Input: part model. Units: mm. Frame: model coordinates. Face numbers are marked on the shaded views. A direction names the side the tool comes from. Coordinates: 2 decimals unless noted, no trailing zeros. Order: outer loops, then holes, each group sorted by start corner. A loop starts at its lowest first (then second) coordinate and runs counter-clockwise, first axis right, second up. Notation, with made-up numbers: (66, 52.5) -> (116, 52.5) arc R31 cw to (116, 80.5) -> close; hole circle Ø7 at (-14.75, 62). An arc over 180 degrees is marked (long way). Answer as CSV lines item,"result".
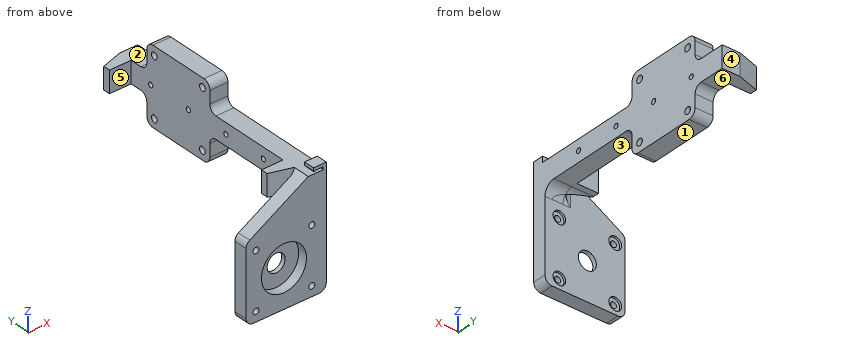
from build123d import *

# Parameters (mm, degrees)
SKETCH1_W           = 42
SKETCH1_H           = 42
SKETCH1_R           = 1.9
BOSS_EXTRUDE1_DEPTH = 10
SKETCH2_W           = 12
SKETCH2_H           = 118
BOSS_EXTRUDE2_DEPTH = 10
SKETCH3_W           = 12
SKETCH3_H           = 3.75
BOSS_EXTRUDE3_DEPTH = 12
CHAMFER1_SIZE       = 3.75
CHAMFER1_SIZE_2     = 12.265697319
SKETCH4_R           = 1.375
CUT_EXTRUDE1_DEPTH  = 12
SKETCH5_W           = 42
SKETCH5_H           = 42
SKETCH5_R           = 1.65
SKETCH5_R_2         = 5
BOSS_EXTRUDE4_DEPTH = 7.5
SKETCH6_R           = 12.5
CUT_EXTRUDE2_DEPTH  = 5.2
FILLET1_R           = 4
FILLET2_R           = 6
SKETCH8_R           = 3.5
CUT_EXTRUDE4_DEPTH  = 1.2
BOSS_EXTRUDE7_DEPTH = 6


with BuildPart() as part:
    # Sketch1 → Boss-Extrude1 (new body)
    with BuildSketch(Plane(origin=(0, 0, 0), x_dir=(0, 0, -1), z_dir=(1, 0, 0))):
        Rectangle(SKETCH1_W, SKETCH1_H)
        with Locations((16, -16)):
            Circle(SKETCH1_R, mode=Mode.SUBTRACT)
        with Locations((-16, -16)):
            Circle(SKETCH1_R, mode=Mode.SUBTRACT)
        with Locations((-16, 16)):
            Circle(SKETCH1_R, mode=Mode.SUBTRACT)
        with Locations((16, 16)):
            Circle(SKETCH1_R, mode=Mode.SUBTRACT)
    extrude(amount=BOSS_EXTRUDE1_DEPTH)

    # Sketch2 → Boss-Extrude2 (add)
    with BuildSketch(Plane.ZY):
        with Locations((0, -20)):
            Rectangle(SKETCH2_W, SKETCH2_H)
    extrude(amount=-BOSS_EXTRUDE2_DEPTH)

    # Sketch3 → Boss-Extrude3 (add)
    with BuildSketch(Plane.ZY):
        with Locations((0, 33.375)):
            Rectangle(SKETCH3_W, SKETCH3_H)
        with Locations((0, -71.575)):
            Rectangle(SKETCH3_W, SKETCH3_H)
    extrude(amount=BOSS_EXTRUDE3_DEPTH)

    # Chamfer1
    # the kernel refuses this chamfer: 12.265697319, 3.75 mm, written as the material it adds along each edge
    with BuildSketch(Plane(origin=(0, 35.25, -6), x_dir=(0.11964200288050787, 0.9928170985366542, 0), z_dir=(0, 0, 1))) as chamfer1_piece_1_section:
        Polygon((CHAMFER1_SIZE * 0.992817098537, CHAMFER1_SIZE * 0.119642002881), (-CHAMFER1_SIZE_2 * 0.119642002884, CHAMFER1_SIZE_2 * 0.992817098562), (0, 0), align=None)
    chamfer1_piece_1 = extrude(amount=12, mode=Mode.PRIVATE)
    chamfer1_piece_1 = split(chamfer1_piece_1, bisect_by=Plane(origin=(-4.172539525, 39, 0), z_dir=(0, -1, 0)), keep=Keep.TOP, mode=Mode.PRIVATE)
    chamfer1_piece_1 = split(chamfer1_piece_1, bisect_by=Plane(origin=(-12, 36.383581674, 0), z_dir=(1, 0, 0)), keep=Keep.TOP, mode=Mode.PRIVATE)
    add(chamfer1_piece_1)
    with BuildSketch(Plane(origin=(0, -73.45, -6), x_dir=(0.11964200288050787, -0.9928170985366542, 0), z_dir=(0, 0, 1))) as chamfer1_piece_2_section:
        Polygon((CHAMFER1_SIZE * 0.992817098537, -CHAMFER1_SIZE * 0.119642002881), (-CHAMFER1_SIZE_2 * 0.119642002884, -CHAMFER1_SIZE_2 * 0.992817098562), (0, 0), align=None)
    chamfer1_piece_2 = extrude(amount=12, mode=Mode.PRIVATE)
    chamfer1_piece_2 = split(chamfer1_piece_2, bisect_by=Plane(origin=(-12, -74.58994207, 0), z_dir=(1, 0, 0)), keep=Keep.TOP, mode=Mode.PRIVATE)
    add(chamfer1_piece_2)

    # Sketch4 → Cut-Extrude1 (cut)
    with BuildSketch(Plane.ZY):
        with Locations((0, 18.4)):
            Circle(SKETCH4_R)
        with Locations((0, -6.6)):
            Circle(SKETCH4_R)
        with Locations((0, -31.6)):
            Circle(SKETCH4_R)
        with Locations((0, -56.6)):
            Circle(SKETCH4_R)
    extrude(amount=-CUT_EXTRUDE1_DEPTH, mode=Mode.SUBTRACT)

    # Sketch5 → Boss-Extrude4 (add)
    # profile 1 of 2: a face of its own
    with BuildSketch(Plane.XZ.offset(79)):
        Polygon((10, -56), (10, 6), (0, 6), (-34.5, -14), (7.5, -14), (7.5, -56), align=None)
    # profile 2 of 2: a face of its own
    with BuildSketch(Plane.XZ.offset(79)):
        with Locations((-13.5, -35)):
            Rectangle(SKETCH5_W, SKETCH5_H)
        with Locations(Location((-29, -50.5, 0), (0, 0, 270))):
            Circle(SKETCH5_R, mode=Mode.SUBTRACT)
        with Locations(Location((-13.5, -35, 0), (0, 0, 270))):
            Circle(SKETCH5_R_2, mode=Mode.SUBTRACT)
        with Locations(Location((2, -50.5, 0), (0, 0, 270))):
            Circle(SKETCH5_R, mode=Mode.SUBTRACT)
        with Locations(Location((-29, -19.5, 0), (0, 0, 270))):
            Circle(SKETCH5_R, mode=Mode.SUBTRACT)
        with Locations(Location((2, -19.5, 0), (0, 0, 270))):
            Circle(SKETCH5_R, mode=Mode.SUBTRACT)
    extrude(amount=BOSS_EXTRUDE4_DEPTH)

    # Sketch6 → Cut-Extrude2 (cut)
    with BuildSketch(Plane.XZ.offset(86.5)):
        with Locations(Location((-13.5, -35, 0), (0, 0, 270))):
            Circle(SKETCH6_R)
    extrude(amount=-CUT_EXTRUDE2_DEPTH, mode=Mode.SUBTRACT)

    # Fillet1
    fillet1_edges = [part.edges().sort_by_distance(p)[0] for p in [
        (-34.5, -82.75, -56),
        (10, -82.75, -56),
        (-34.5, -82.75, -14),
        (5, -21, 6),
        (5, -21, -6),
        (5, 21, -6),
        (5, 21, 6),
        (5, -21, -21),
        (5, -21, 21),
        (5, 21, 21),
        (5, 21, -21),
    ]]
    fillet(fillet1_edges, radius=FILLET1_R)

    # Fillet2
    # the kernel refuses this fillet: 6 mm, written as the material it adds along each edge
    with BuildSketch(Plane(origin=(0, -79, -6), x_dir=(0, 1, 0), z_dir=(1, 0, 0))) as fillet2_piece_1_section:
        with BuildLine():
            CenterArc((FILLET2_R, -FILLET2_R), FILLET2_R, 90, 90)
            Line((0, -FILLET2_R), (-FILLET2_R * 0.02, -FILLET2_R))
            Line((-FILLET2_R * 0.02, -FILLET2_R), (-FILLET2_R * 0.02, FILLET2_R * 0.02))
            Line((-FILLET2_R * 0.02, FILLET2_R * 0.02), (FILLET2_R, FILLET2_R * 0.02))
            Line((FILLET2_R, FILLET2_R * 0.02), (FILLET2_R, 0))
        make_face()
    fillet2_piece_1 = extrude(amount=10, mode=Mode.PRIVATE)
    fillet2_piece_1 = split(fillet2_piece_1, bisect_by=Plane(origin=(2.499298027, -77.964112089, -8.062690797), z_dir=(-0.29237170472287155, -0.9563047559629945, 0)), keep=Keep.TOP, mode=Mode.PRIVATE)
    add(fillet2_piece_1)
    with BuildSketch(Plane(origin=(-15, -79, -6), x_dir=(0, 1, 0), z_dir=(1, 0, 0))) as fillet2_piece_2_section:
        with BuildLine():
            CenterArc((FILLET2_R, -FILLET2_R), FILLET2_R, 90, 90)
            Line((0, -FILLET2_R), (-FILLET2_R * 0.02, -FILLET2_R))
            Line((-FILLET2_R * 0.02, -FILLET2_R), (-FILLET2_R * 0.02, FILLET2_R * 0.02))
            Line((-FILLET2_R * 0.02, FILLET2_R * 0.02), (FILLET2_R, FILLET2_R * 0.02))
            Line((FILLET2_R, FILLET2_R * 0.02), (FILLET2_R, 0))
        make_face()
    fillet2_piece_2 = extrude(amount=25, mode=Mode.PRIVATE)
    fillet2_piece_2 = split(fillet2_piece_2, bisect_by=Plane(origin=(-12, -75.195203729, -6.203668613), z_dir=(1, 0, 0)), keep=Keep.TOP, mode=Mode.PRIVATE)
    fillet2_piece_2 = split(fillet2_piece_2, bisect_by=Plane(origin=(-3.530108064, -76.120737656, -6.203668613), z_dir=(0.29237170472287155, 0.9563047559629945, 0)), keep=Keep.TOP, mode=Mode.PRIVATE)
    fillet2_piece_2 = split(fillet2_piece_2, bisect_by=Plane(origin=(0, -75.195203729, -6.203668613), z_dir=(-1, 0, 0)), keep=Keep.TOP, mode=Mode.PRIVATE)
    add(fillet2_piece_2)
    with BuildSketch(Plane(origin=(0, -79, -6), x_dir=(0, 1, 0), z_dir=(1, 0, 0))) as fillet2_piece_3_section:
        with BuildLine():
            CenterArc((FILLET2_R, -FILLET2_R), FILLET2_R, 90, 90)
            Line((0, -FILLET2_R), (-FILLET2_R * 0.02, -FILLET2_R))
            Line((-FILLET2_R * 0.02, -FILLET2_R), (-FILLET2_R * 0.02, FILLET2_R * 0.02))
            Line((-FILLET2_R * 0.02, FILLET2_R * 0.02), (FILLET2_R, FILLET2_R * 0.02))
            Line((FILLET2_R, FILLET2_R * 0.02), (FILLET2_R, 0))
        make_face()
    fillet2_piece_3 = extrude(amount=10, mode=Mode.PRIVATE)
    fillet2_piece_3 = split(fillet2_piece_3, bisect_by=Plane(origin=(5.482207423, -78.876079011, -7.106323333), z_dir=(0.29237170472287155, 0.9563047559629945, 0)), keep=Keep.TOP, mode=Mode.PRIVATE)
    add(fillet2_piece_3)
    with BuildSketch(Plane(origin=(0, -79, -6), x_dir=(-1, 0, 0), z_dir=(0, 0, 1))) as fillet2_piece_4_section:
        with BuildLine():
            CenterArc((4.284857057, -6), FILLET2_R, 90, 45.572995999)
            Line((0, -1.8), (-0.085697141, -1.716))
            ThreePointArc((-0.085697141, -1.716), (-0.12, -0.9), (-0.12, 0))
            Line((-0.12, 0), (0, 0.12))
            Line((0, 0.12), (4.284857057, 0.12))
            Line((4.284857057, 0.12), (4.284857057, 0))
        make_face()
    fillet2_piece_4 = extrude(amount=12, mode=Mode.PRIVATE)
    fillet2_piece_4 = split(fillet2_piece_4, bisect_by=Plane(origin=(-3.559533533, -78.541465105, 3.936502299), z_dir=(0.5015304356318926, 0, -0.8651400014650138)), keep=Keep.TOP, mode=Mode.PRIVATE)
    add(fillet2_piece_4)
    with BuildSketch(Plane(origin=(-15, -79, -6), x_dir=(0, 1, 0), z_dir=(1, 0, 0))) as fillet2_piece_5a_section:
        with BuildLine():
            CenterArc((FILLET2_R, -FILLET2_R), FILLET2_R, 90, 90)
            Line((0, -FILLET2_R), (-FILLET2_R * 0.02, -FILLET2_R))
            Line((-FILLET2_R * 0.02, -FILLET2_R), (-FILLET2_R * 0.02, FILLET2_R * 0.02))
            Line((-FILLET2_R * 0.02, FILLET2_R * 0.02), (FILLET2_R, FILLET2_R * 0.02))
            Line((FILLET2_R, FILLET2_R * 0.02), (FILLET2_R, 0))
        make_face()
    fillet2_piece_5a = extrude(amount=25, mode=Mode.PRIVATE)
    fillet2_piece_5a = split(fillet2_piece_5a, bisect_by=Plane(origin=(-12, -77.909616739, -7.484859566), z_dir=(1, 0, 0)), keep=Keep.TOP, mode=Mode.PRIVATE)
    fillet2_piece_5a = split(fillet2_piece_5a, bisect_by=Plane(origin=(-5.56448371, -75.498766603, -7.484859566), z_dir=(-0.29237170472287155, -0.9563047559629945, 0)), keep=Keep.TOP, mode=Mode.PRIVATE)
    fillet2_piece_5a = split(fillet2_piece_5a, bisect_by=Plane(origin=(0, -77.909616739, -7.484859566), z_dir=(-1, 0, 0)), keep=Keep.TOP, mode=Mode.PRIVATE)
    with BuildSketch(Plane(origin=(0, -79, -16.712142643), x_dir=(-1, 0, 0), z_dir=(0, 0, 1))) as fillet2_piece_5b_section:
        with BuildLine():
            CenterArc((4.284857057, -6), FILLET2_R, 90, 45.572995999)
            Line((0, -1.8), (-0.085697141, -1.716))
            ThreePointArc((-0.085697141, -1.716), (-0.12, -0.9), (-0.12, 0))
            Line((-0.12, 0), (0, 0.12))
            Line((0, 0.12), (4.284857057, 0.12))
            Line((4.284857057, 0.12), (4.284857057, 0))
        make_face()
    fillet2_piece_5b = extrude(amount=22.712142643, mode=Mode.PRIVATE)
    fillet2_piece_5b = split(fillet2_piece_5b, bisect_by=Plane(origin=(-1.145977821, -78.554932171, -6), z_dir=(0, 0, -1)), keep=Keep.TOP, mode=Mode.PRIVATE)
    fillet2_piece_5 = fillet2_piece_5a & fillet2_piece_5b
    add(fillet2_piece_5)

    # Sketch8 → Cut-Extrude4 (cut)
    with BuildSketch(Plane(origin=(0, -79, 0), x_dir=(1, 0, 0), z_dir=(0, 1, 0))):
        with Locations(Location((-29, 50.5, 0), (0, 0, 270))):
            Circle(SKETCH8_R)
        with Locations(Location((2, 50.5, 0), (0, 0, 270))):
            Circle(SKETCH8_R)
        with Locations(Location((2, 19.5, 0), (0, 0, 270))):
            Circle(SKETCH8_R)
        with Locations(Location((-29, 19.5, 0), (0, 0, 270))):
            Circle(SKETCH8_R)
    extrude(amount=-CUT_EXTRUDE4_DEPTH, mode=Mode.SUBTRACT)

    # Sketch11 → Boss-Extrude7 (add)
    with BuildSketch(Plane.XZ.offset(86.5)):
        Polygon((8.3, 6), (10, 6), (10, 9.2), (2.9, 9.2), (2.9, 7.5), (3.9, 7.5), (8.3, 7.5), align=None)
        Polygon((3.9, 7.5), (2.9, 7.5), (3.433368825, 6.8), align=None)
    extrude(amount=-BOSS_EXTRUDE7_DEPTH)


solid = part.part
1. Reachability of the marked faces 1, 2 and 3 from +Z, -Z, +X, -X, +Y, -Y: full face, straight path, thin tool, end or side. Return the list, or none.
Findings:
face 1,"-Z, +X, -X, +Y"
face 2,"+Z, +X, -X, +Y"
face 3,"-Z, +X, -X"
2. Contact query for flat-ended pins moving along their axis: pin 1 (8 mm diameter, centred on x = 4, z = -7.5, fed in from +Y); pin 2 (2 mm diameter, centred on x = 2.5, z = 15, fed in from -Y); pin 3 (12 mm diameter, centred on x = 4.5, y = -48.5, fed in from +Z); pin 4 (2.5 mm diameter, centred on y = 16, z = 16, fed in from +X). Output: stop coordinate, or through.
Findings:
pin 1,"stops at y = 39"
pin 2,"stops at y = -21"
pin 3,"stops at z = 6"
pin 4,"passes through"
3. Ray query, line 1 along Y through (x, z) = (3.5, 0) (3 decimals); line 2 along Y through (x, z) = (4, 16); line 3 along Y through (x, z) = (5.5, -17.5). Return the intervals inside material, ascending.
Findings:
line 1,"y = -86.5 to -57.975, -55.225 to -32.975, -30.225 to -7.975, -5.225 to 17.025, 19.775 to 39"
line 2,"y = -21 to -17.9, -14.1 to 14.1, 17.9 to 21"
line 3,"y = -86.5 to -79, -20.97 to -17.17, -14.83 to 14.83, 17.17 to 20.97"
4. Cut plane C-C (z = -50.5). Return the cut outline in (x, y).
Findings:
outline,"(-34.5, -86.5) -> (-30.65, -86.5) -> (-30.65, -80.2) -> (-32.5, -80.2) -> (-32.5, -79) -> (-34.5, -79) -> close; (-27.35, -86.5) -> (0.35, -86.5) -> (0.35, -80.2) -> (-1.5, -80.2) -> (-1.5, -79) -> (-25.5, -79) -> (-25.5, -80.2) -> (-27.35, -80.2) -> close; (3.65, -86.5) -> (10, -86.5) -> (10, -79) -> (5.5, -79) -> (5.5, -80.2) -> (3.65, -80.2) -> close"
5. Cut plane D-D (x = -13.5). Return the cut outline in (y, z), plus the area to 3 significant figures.
Findings:
outline,"(-86.5, -56) -> (-79, -56) -> (-79, -40) -> (-81.3, -40) -> (-81.3, -47.5) -> (-86.5, -47.5) -> close; (-86.5, -22.5) -> (-81.3, -22.5) -> (-81.3, -30) -> (-79, -30) -> (-79, -1.83) -> (-86.5, -1.83) -> close"
area,"253 mm2"
6. Mould query, pull axis Y, two halves, no side actions, for the marked faces 4, 5 and 6. Classes: released by +Y, released by -Y, zero draft, split by the parting line, or undercut.
Findings:
face 4,"released by +Y"
face 5,"undercut"
face 6,"zero draft"
7. Cut plane A-A (y = -56.6). Return the cut outline in (x, z) (3 decimals), plus the area to 3 significant figures.
Findings:
outline,"(0, -6) -> (10, -6) -> (10, -1.375) -> (0, -1.375) -> close; (0, 1.375) -> (10, 1.375) -> (10, 6) -> (0, 6) -> close"
area,"92.5 mm2"
8. Cut plane B-B (z = -35). Return the cut outline in (x, y), plus the area to 3 significant figures.
Findings:
outline,"(-34.5, -86.5) -> (-26, -86.5) -> (-26, -81.3) -> (-18.5, -81.3) -> (-18.5, -79) -> (-34.5, -79) -> close; (-8.5, -81.3) -> (-1, -81.3) -> (-1, -86.5) -> (10, -86.5) -> (10, -79) -> (-8.5, -79) -> close"
area,"181 mm2"
